Geometry: see drawing. Coordinates: mm, zero at the bounding-box minimum. A direction names the side the tool comes from. Give positions to 0.01 mm unless a question says otherwise; leave off trailing zeros. Loops run counter-clockwise (first coordinate to the right, second up) from the corner with the lowest first, then second, coordinate; pieces in that order, holes last. Notation, with made-up numbers: M 13,-36.75 L 24,-36.75 A12 cw 24,-26.75 Z; hole C 0.25,81.25 d2. An arc over 180 degrees is marked long. Put each result on its own line as item: value.
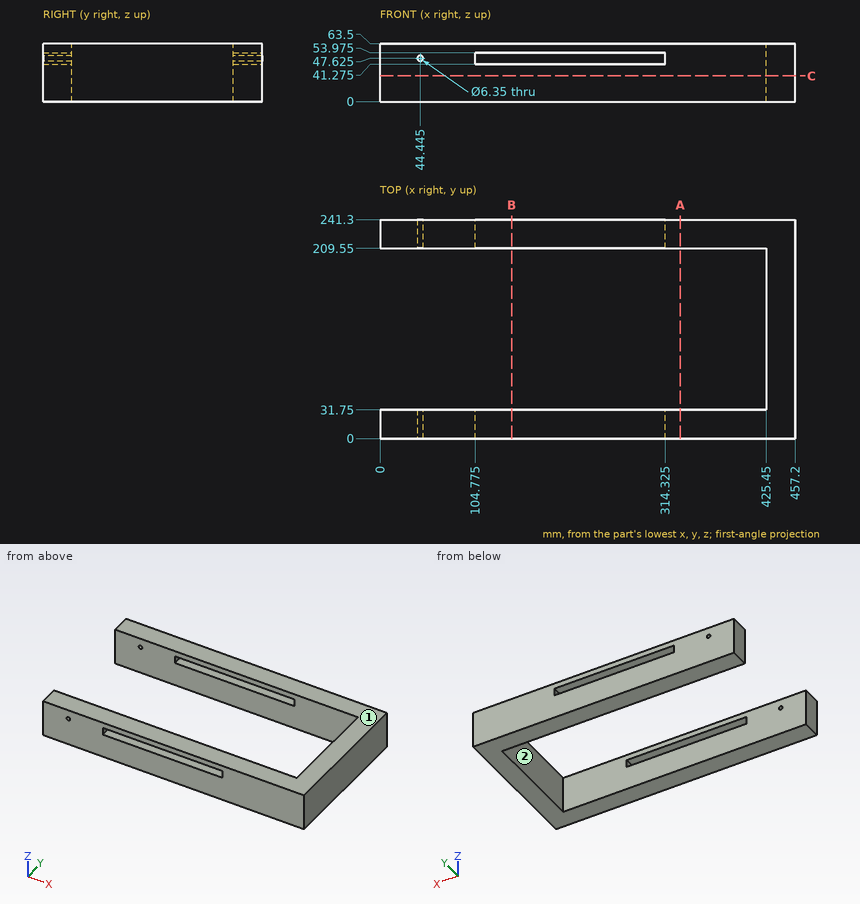
1. Section query C-C (z = 28.5). Output: boundary loops of the cut face in (x, y), plus the area to 3 significant figures.
Found:
outline: M 0,0 L 457.2,0 L 457.2,241.3 L 0,241.3 L 0,209.55 L 425.45,209.55 L 425.45,31.75 L 0,31.75 Z
area: 34,700 mm^2
2. Section query A-A (x = 331). Output: boundary loops of the cut face in (y, z), plus the area to 3 significant figures.
Found:
outline: M 0,0 L 31.75,0 L 31.75,63.5 L 0,63.5 Z; M 209.55,0 L 241.3,0 L 241.3,63.5 L 209.55,63.5 Z
area: 4,030 mm^2
3. Section query B-B (x = 145). State how many separate pieces and enclosed holes the cut face has, plus the area to 3 significant figures.
Found:
separate pieces: 4
enclosed holes: 0
area: 3,230 mm^2
4. Access query for the marked faces 1 and 2. Directions: +Z, -Z, +X, -X, +Y, -Y. A direction counts if a zero-diameter tool reaches every point of the face in a straight line with its end or side. Return the directions, or none.
Found:
face 1: +Z, +X, -X, +Y, -Y
face 2: +Z, -Z, -X
5. Material intervals for line 1 (Y direction, x = 219, z = 28.5); line 2 (X direction, y = 66, z = 52), sorted ascending. Write a range as from..to.
Found:
line 1: 0..31.75, 209.55..241.3
line 2: 425.45..457.2
